The model under review builds one solid part; all positions refer to its coordinate system, in mm. A direction names the side the tool comes from. Round coordinates to 2 decimals unless told otherwise and drop trailing zeros. Loops run counter-clockwise (first coordinate to the right, second up) from the corner with the lowest first, then second, coordinate; pieces in that order, holes last. Notation, with made-up numbers: (59.25, 12.5) -> (117.25, 12.5) arc R8 cw to (117.25, 26.5) -> close; hole circle Ø1 at (66, 59.5). An arc over 180 degrees is marked (long way). Use a Markdown table: item, result. Add a question column.
1) Consider section C-C on z = -44. Give the boundary of the cut face in (x, y), plus the area to 3 significant figures.
2) Insertion check: pin 1 (14 mm diameter, centred on x = -8, z = -49.5, fed in from -Y). The pin has a flat end and moves straight along its axis. Give the tip position at first contact, or say it passes through.
3) Wall thickness on probe 1 along X at (y, z) = (-37, -56.5); probe 2 along Y at (x, z) = (-23, -47.75); probe 3 along Y at (x, z) = (-8, -56.5): over which ranges is each line inside the solid? List them lowest first.
4) For faces 5 (the flat face through (-9, -62.301, -52)), 6 (the flat face through (-30, -29.281, -52)), 7 (the flat face through (-34, 3.739, -52)), list the 3-axis set-ups (+Z, -Z, +X, -X, +Y, -Y) from which the entire face can be reached by the end or side of a thin tool; tool diameter is ignored.
5) Consider section B-B on y = -46. Give the boundary of the cut face in (x, z), plus the area to 3 significant figures.
6) Mouldability with a two-part tool opening along X and no side actions: class faces 1 (the flat face through (-44, -80.081, -52)), 2 (the flat face through (-17.755, -71, -52)), 3 (the flat face through (-43.18, -46, -52)), 4 (the flat face through (-17.78, -46, -52)) as released by +X, released by -X, zero draft, split by the parting line, or undercut.
7) Consider section A-A on x = -20.5. Give the boundary of the cut face in (y, z).
from build123d import *

# Parameters (mm, degrees)
F0_W     = 33.02
F0_H     = 25.4
F1_DEPTH = 17.78
F2_DEPTH = 68.58
F3_W     = 25.4
F3_H     = 25.4
F4_DEPTH = 50.8
F5_W     = 17.78
F5_H     = 25.4
F6_DEPTH = 25.4254


with BuildPart() as f1:
    # F0 (on Right) → F1 (new body)
    with BuildSketch(Plane.YZ):
        with Locations((-45.790768, -52.245537)):
            Rectangle(F0_W, F0_H)
    extrude(amount=-F1_DEPTH)

    # F0 (on Right) → F2 (join)
    with BuildSketch(Plane.YZ):
        with Locations((-12.770768, -52.245537)):
            Rectangle(F0_W, F0_H)
    extrude(amount=-F2_DEPTH)

    # F3 (on face) → F4 (join)
    with BuildSketch(Plane.XZ.offset(29.280768)):
        with Locations((-55.88, -52.245537)):
            Rectangle(F3_W, F3_H)
    extrude(amount=F4_DEPTH)

    # F5 (on face) → F6 (join)
    with BuildSketch(Plane.YZ.offset(-43.18)):
        with Locations((-71.190768, -52.245537)):
            Rectangle(F5_W, F5_H)
    extrude(amount=F6_DEPTH)


solid = f1.part
Result set:
| question | item | result |
|---|---|---|
| 1 | outline | (-68.58, -80.08) -> (-17.75, -80.08) -> (-17.75, -62.3) -> (0, -62.3) -> (0, 3.74) -> (-68.58, 3.74) -> close; hole (-43.18, -62.3) -> (-17.78, -62.3) -> (-17.78, -29.28) -> (-43.18, -29.28) -> close |
| 1 | area | 4,590 mm2 |
| 2 | pin 1 | y = -62.3 |
| 3 | probe 1 | -68.58 to -43.18, -17.78 to 0 |
| 3 | probe 2 | -80.08 to -62.3, -29.28 to 3.74 |
| 3 | probe 3 | -62.3 to 3.74 |
| 4 | face 5 | +Z, -Z, +X, -Y |
| 4 | face 6 | +Z, -Z |
| 4 | face 7 | +Z, -Z, +X, -X, +Y |
| 5 | outline | (-68.58, -64.95) -> (-43.18, -64.95) -> (-43.18, -39.55) -> (-68.58, -39.55) -> close; (-17.78, -64.95) -> (0, -64.95) -> (0, -39.55) -> (-17.78, -39.55) -> close |
| 5 | area | 1,100 mm2 |
| 6 | face 1 | zero draft |
| 6 | face 2 | released by +X |
| 6 | face 3 | undercut |
| 6 | face 4 | undercut |
| 7 | outline | (-80.08, -64.95) -> (-62.3, -64.95) -> (-62.3, -39.55) -> (-80.08, -39.55) -> close; (-29.28, -64.95) -> (3.74, -64.95) -> (3.74, -39.55) -> (-29.28, -39.55) -> close |
